Could you check a few things on this model? Use its own coordinates, in mm. Coordinates: 2 decimals unless noted, no trailing zeros. Loops run counter-clockwise (first coordinate to the right, second up) from the corner with the lowest first, then second, coordinate; pieces in that order, holes last.
from build123d import *

# Parameters (mm, degrees)
BOSS_EXTRUDE1_DEPTH = 42
SKETCH2_R           = 12
SKETCH2_R_2         = 1.5
CUT_EXTRUDE1_DEPTH  = 5
SKETCH3_R           = 2
CUT_EXTRUDE2_DEPTH  = 5
CHAMFER1_SIZE       = 2
CHAMFER2_SIZE       = 1
FILLET1_R           = 4
BOSS_EXTRUDE2_DEPTH = 42
SKETCH5_W           = 27.168576179
SKETCH5_H           = 4
CUT_EXTRUDE3_DEPTH  = 44
SKETCH6_R           = 2.5
CUT_EXTRUDE4_DEPTH  = 44
FILLET2_R           = 4


with BuildPart() as part:
    # Sketch1 → Boss-Extrude1 (new body)
    with BuildSketch(Plane(origin=(0, 0, 0), x_dir=(1, 0, 0), z_dir=(0, 1, 0))):
        Polygon((0, 0), (0, 42), (-20, 42), (-20, 46), (4, 46), (4, 0), align=None)
    extrude(amount=BOSS_EXTRUDE1_DEPTH)

    # Sketch2 → Cut-Extrude1 (cut, through all)
    with BuildSketch(Plane.ZY):
        with Locations((-21, 21)):
            Circle(SKETCH2_R)
        with Locations((-36.5, 36.5)):
            Circle(SKETCH2_R_2)
        with Locations((-5.5, 36.5)):
            Circle(SKETCH2_R_2)
        with Locations((-5.5, 5.5)):
            Circle(SKETCH2_R_2)
        with Locations((-36.5, 5.5)):
            Circle(SKETCH2_R_2)
    extrude(amount=-CUT_EXTRUDE1_DEPTH, mode=Mode.SUBTRACT)

    # Sketch3 → Cut-Extrude2 (cut, through all)
    with BuildSketch(Plane.XY.offset(-42)):
        with Locations((-10, 32)):
            Circle(SKETCH3_R)
        with Locations((-10, 10)):
            Circle(SKETCH3_R)
    extrude(amount=-CUT_EXTRUDE2_DEPTH, mode=Mode.SUBTRACT)

    # Chamfer1
    chamfer1_edges = [part.edges().sort_by_distance(p)[0] for p in [
        (-12, 32, -42),
        (-12, 10, -42),
    ]]
    chamfer(chamfer1_edges, length=CHAMFER1_SIZE)

    # Chamfer2
    chamfer2_edges = [part.edges().sort_by_distance(p)[0] for p in [
        (0, 21, -33),
    ]]
    chamfer(chamfer2_edges, length=CHAMFER2_SIZE)

    # Fillet1
    fillet1_edges = [part.edges().sort_by_distance(p)[0] for p in [
        (4, 21, -46),
        (-20, 42, -44),
        (2, 42, 0),
        (-20, 0, -44),
        (2, 0, 0),
    ]]
    fillet(fillet1_edges, radius=FILLET1_R)

    # Sketch4 → Boss-Extrude2 (add)
    with BuildSketch(Plane.XZ):
        Polygon((0, -46), (0, -66), (4, -66), (4, -42), (0, -42), align=None)
    extrude(amount=-BOSS_EXTRUDE2_DEPTH)

    # Sketch5 → Cut-Extrude3 (cut)
    with BuildSketch(Plane(origin=(0, 42, 0), x_dir=(1, 0, 0), z_dir=(0, 1, 0))):
        with Locations((-13.58428809, 44)):
            Rectangle(SKETCH5_W, SKETCH5_H)
    extrude(amount=-CUT_EXTRUDE3_DEPTH, mode=Mode.SUBTRACT)

    # Sketch6 → Cut-Extrude4 (cut)
    with BuildSketch(Plane.ZY):
        with Locations((-56, 32)):
            Circle(SKETCH6_R)
        with Locations((-56, 10)):
            Circle(SKETCH6_R)
    extrude(amount=-CUT_EXTRUDE4_DEPTH, mode=Mode.SUBTRACT)

    # Fillet2
    fillet2_edges = [part.edges().sort_by_distance(p)[0] for p in [
        (2, 42, -66),
        (2, 0, -66),
    ]]
    fillet(fillet2_edges, radius=FILLET2_R)


solid = part.part
(1) For pin 1 (21.5 mm diameter, centred on y = 21, z = -21, fed in from +X), with a flat end and sliding along its axis, tell me the tip position at first contact or that it passes through.
Answers:
pin 1: passes through
(2) Imagine slicing it at C-C, the plane z = -21. Write out the boundary of the cut face in (x, y), and give its area (3 significant figures).
Answers:
outline: (0, 0) - (4, 0) - (4, 9) - (1, 9) - (0, 8) - close; (0, 34) - (1, 33) - (4, 33) - (4, 42) - (0, 42) - close
area: 71.0 mm2
(3) Imagine slicing it at B-B, the plane z = -5.5. Write out the boundary of the cut face in (x, y), and give its area (3 significant figures).
Answers:
outline: (0, 0) - (4, 0) - (4, 4) - (0, 4) - close; (0, 7) - (4, 7) - (4, 35) - (0, 35) - close; (0, 38) - (4, 38) - (4, 42) - (0, 42) - close
area: 144 mm2
(4) I need wall thicknesses on probe 1 along Y at (x, z) = (2.5, -36.5); probe 2 along Z at (x, y) = (1.7, 31); probe 3 along Z at (x, y) = (2.25, 35.5). Which ranges of each line are inside material? Lowest first, please.
Answers:
probe 1: y = 0 to 4, 7 to 35, 38 to 42
probe 2: z = -66 to -58.29, -53.71 to -27.63, -14.37 to 0
probe 3: z = -66 to -37.62, -35.38 to -6.62, -4.38 to 0
(5) Imagine slicing it at D-D, the plane y = 21. Write out the boundary of the cut face in (x, z).
Answers:
outline: (0, -66) - (4, -66) - (4, -33) - (1, -33) - (0, -34) - close; (0, -8) - (1, -9) - (4, -9) - (4, 0) - (0, 0) - close
(6) Imagine slicing it at A-A, the plane y = 36.5. Write out the boundary of the cut face in (x, z), and give its area (3 significant figures).
Answers:
outline: (0, -66) - (4, -66) - (4, -38) - (0, -38) - close; (0, -35) - (4, -35) - (4, -7) - (0, -7) - close; (0, -4) - (4, -4) - (4, 0) - (0, 0) - close
area: 240 mm2
(7) We'd pull the mould along Y, two halves only. Please class faces 1 (the face through (1.97, 34.11, -54.66)), 2 (the face through (1.972, 1.203, -1.141)), 3 (the face through (1.972, 35.036, -5.825)), 4 (the face through (1.972, 40.797, -1.141)): +Y half, -Y half, draft (parallel to the pull), parting line (faces both ways), or undercut.
Answers:
face 1: undercut
face 2: -Y half
face 3: undercut
face 4: +Y half
